Verification items for this drawing (mm, ordinates from the low corner). Coordinates: 2 decimals unless noted, no trailing zeros. Write each loop counter-clockwise with the first axis right and the second up, starting at its lowest first coordinate (ties: lowest second). Pieces come first, ordered by that corner, then holes. Notation, with made-up numbers: (-2, -37) -> (56, -37) arc R34 ccw to (56, -1) -> close; hole circle Ø10 at (48, 40.25). An arc over 180 degrees is marked (long way). Answer as CSV lines item,"result".
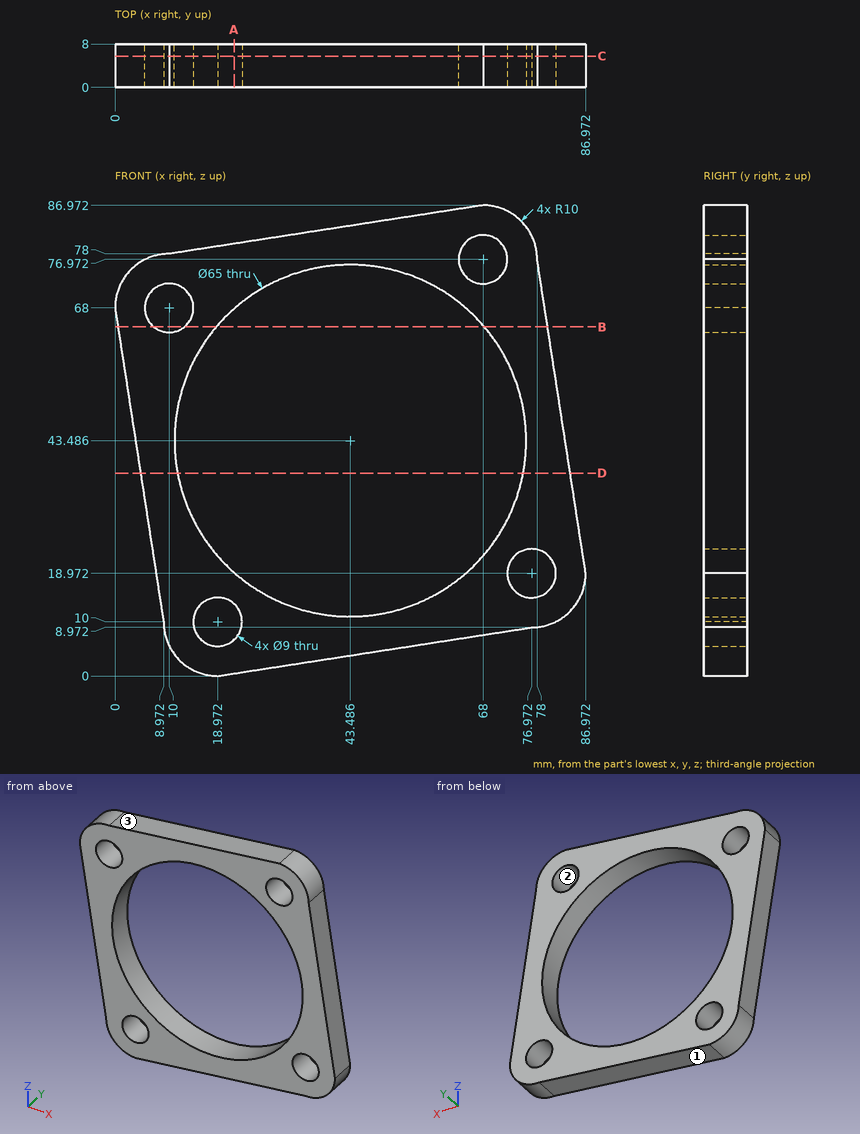
Item 1: Cross-section at D-D, the plane z = 37.5. Record the cut outline in (x, y), plus the area to 3 significant figures.
Responses:
outline,"(4.72, 0) -> (11.54, 0) -> (11.54, 8) -> (4.72, 8) -> close; (75.43, 0) -> (84.11, 0) -> (84.11, 8) -> (75.43, 8) -> close"
area,"124 mm2"
Item 2: Depth check by flat-ended pin: pin 1 Ø5.5 at (x, z) = (18.97, 10) entering from -Y; pin 2 Ø4 at (y, z) = (3.5, 11) entering from -X; pin 3 Ø2 at (y, z) = (3.5, 33.5) entering from -X; pin 4 Ø2 at (y, z) = (6.5, 25) entering from +X. Enter the tip coordinate at first touch or a pass-through.
Responses:
pin 1,"passes through"
pin 2,"stops at x = 8.51"
pin 3,"stops at x = 5.18"
pin 4,"stops at x = 86.19"
Item 3: Cross-section at A-A, the plane x = 22. Record the cut outline in (y, z), plus the area to 3 significant figures.
Responses:
outline,"(0, 0.47) -> (8, 0.47) -> (8, 6.67) -> (0, 6.67) -> close; (0, 13.33) -> (8, 13.33) -> (8, 19.1) -> (0, 19.1) -> close; (0, 67.87) -> (8, 67.87) -> (8, 79.86) -> (0, 79.86) -> close"
area,"192 mm2"
Item 4: Thickness scan on probe 1 along Z at (x, y) = (16, 1.75) (1 decimal); probe 2 along Z at (x, y) = (22, 1.25); probe 3 along X at (y, z) = (2.75, 18) (1 decimal). Record the ranges inside material, lowest first.
Responses:
probe 1,"z = 0.5 to 6.6, 13.4 to 26.1, 60.8 to 78.9"
probe 2,"z = 0.47 to 6.67, 13.33 to 19.1, 67.87 to 79.86"
probe 3,"x = 7.7 to 23.3, 63.7 to 72.6, 81.4 to 86.9"
Item 5: Release check for a two-part mould opening along X. For the marked faces 1, 2 and 3 record: +X half, -X half, draft (parallel to the pull), parting line (faces both ways), or undercut.
Responses:
face 1,"+X half"
face 2,"undercut"
face 3,"-X half"
Item 6: Cross-section at C-C, the plane y = 5.75. Record the cut outline in (x, z), plus the area to 3 significant figures.
Responses:
outline,"(0, 68) -> (8.97, 10) arc R10 ccw to (18.97, 0) -> (76.97, 8.97) arc R10 ccw to (86.97, 18.97) -> (78, 76.97) arc R10 ccw to (68, 86.97) -> (10, 78) arc R10 ccw to start; hole circle Ø9 at (10, 68); hole circle Ø65 at (43.49, 43.49); hole circle Ø9 at (18.97, 10); hole circle Ø9 at (68, 76.97); hole circle Ø9 at (76.97, 18.97)"
area,"2,510 mm2"
Item 7: Cross-section at B-B, the plane z = 64.5. Record the cut outline in (x, y), plus the area to 3 significant figures.
Responses:
outline,"(0.54, 0) -> (7.17, 0) -> (7.17, 8) -> (0.54, 8) -> close; (12.83, 0) -> (18.69, 0) -> (18.69, 8) -> (12.83, 8) -> close; (68.28, 0) -> (79.93, 0) -> (79.93, 8) -> (68.28, 8) -> close"
area,"193 mm2"
